Geometry: final body of the model. Coordinates: model frame, mm. Face numbers are marked on the shaded views. Give positions to 0.01 mm unless a question says otherwise; leave off trailing zeros. Write each loop counter-clockwise with the first axis right and the second up, starting at its lowest first coordinate (ties: lowest second). Pieces come first, ordered by that corner, then holes. Notation, with made-up numbers: M 33.5,-0.75 L 53.5,-0.75 A31 ccw 53.5,36.25 Z; hole C 75,59 d5. An arc over 180 degrees is marked long. Answer as a JSON object with one key per item and string values.
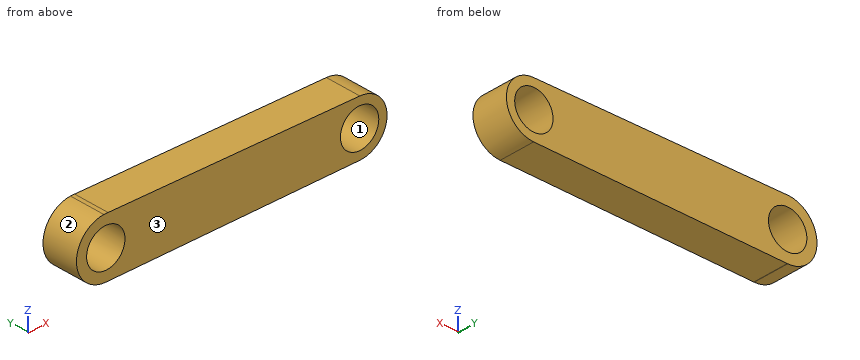
from build123d import *

# Parameters (mm, degrees)
F0_R     = 5.385815
F0_R_2   = 5.385812
F1_DEPTH = 10.16


with BuildPart() as f1:
    # F0 (on Front) → F1 (new body)
    with BuildSketch(Plane.XZ):
        with BuildLine():
            Line((-40.131064, 8.215562), (-38.943939, 8.207193))
            ThreePointArc((-38.943939, 8.207193), (-39.53735, 8.232802), (-40.131064, 8.215562))
        make_face()
        with BuildLine():
            Line((31.730667, 7.708937), (-38.943939, 8.207193))
            Line((-38.943939, 8.207193), (-40.131064, 8.215562))
            ThreePointArc((-40.131064, 8.215562), (-47.824065, -0.267089), (-39.59717, -8.233007))
            Line((-39.59717, -8.233007), (-39.472638, -8.232092))
            Line((-39.472638, -8.232092), (31.732959, -7.70892))
            ThreePointArc((31.732959, -7.70892), (39.385447, 0.001146), (31.730667, 7.708937))
        make_face()
        with Locations((-39.595392, 0)):
            Circle(F0_R, mode=Mode.SUBTRACT)
        with Locations((31.676318, 0)):
            Circle(F0_R_2, mode=Mode.SUBTRACT)
        with BuildLine():
            Line((-39.472638, -8.232092), (-39.59717, -8.233007))
            ThreePointArc((-39.59717, -8.233007), (-39.534903, -8.232785), (-39.472638, -8.232092))
        make_face()
    extrude(amount=F1_DEPTH)


solid = f1.part
1) Line query: line 1 (X direction, y = -8, z = -0.25); line 2 (X direction, y = -7, z = -1.5); line 3 (Z direction, x = -44, y = -9.5). Output: solid intervals per line, ascending. Write a range as from..to.
Geometry check:
{"line 1": "x = -47.82..-44.98, -34.22..26.3, 37.06..39.38", "line 2": "x = -47.69..-44.77, -34.42..26.5, 36.85..39.24", "line 3": "z = -6.96..-3.1, 3.1..6.96"}
2) Contact query for flat-ended pins moving along their axis: P1, Ø8.5, axis at x = -39.6, z = 0, coming from the +Y side; P2, Ø2, axis at y = -4, z = 6, coming from the -X side; P3, Ø8, axis at x = -22.5, z = 0.5, coming from the +Y side; P4, Ø1.5, axis at y = -2, z = -1, coming from the -X side. Output: stop coordinate, or through.
Geometry check:
{"P1": "passes through", "P2": "stops at x = -46.14", "P3": "stops at y = 0", "P4": "stops at x = -47.82"}
3) Cut plane B-B on y = -6.5. Return loops of the section in (x, z), and give its area (3 significant figures).
Geometry check:
{"outline": "M -40.13,8.22 A8.23 ccw -39.6,-8.23 A8.23 ccw -39.47,-8.23 L 31.73,-7.71 A7.71 ccw 31.73,7.71 L -38.94,8.21 A8.23 ccw Z; hole C -39.6,0 d10.77; hole C 31.68,0 d10.77", "area": "1,150 mm2"}
4) Cut plane A-A on z = 0. Return loops of the section in (x, y), and give its area (3 significant figures).
Geometry check:
{"outline": "M -47.83,-10.16 L -44.98,-10.16 L -44.98,0 L -47.83,0 Z; M -34.21,-10.16 L 26.29,-10.16 L 26.29,0 L -34.21,0 Z; M 37.06,-10.16 L 39.39,-10.16 L 39.39,0 L 37.06,0 Z", "area": "667 mm2"}
5) Cut plane D-D on x = 21.5. Return loops of the section in (y, z).
Geometry check:
{"outline": "M -10.16,-7.78 L 0,-7.78 L 0,7.78 L -10.16,7.78 Z"}
6) Cut plane C-C on z = -4. Return loops of the section in (x, y).
Geometry check:
{"outline": "M -46.79,-10.16 L -43.2,-10.16 L -43.2,0 L -46.79,0 Z; M -35.99,-10.16 L 28.07,-10.16 L 28.07,0 L -35.99,0 Z; M 35.28,-10.16 L 38.27,-10.16 L 38.27,0 L 35.28,0 Z"}
7) Pull-direction query (X, two-part tool) for the marked faces 1, 2 and 3; classes: pulls with the +X half, pulls with the -X half, needs draft (parallel to the pull), parting line crosses it, or undercut.
Geometry check:
{"face 1": "undercut", "face 2": "pulls with the -X half", "face 3": "needs draft"}
